The model under review builds one solid part; all positions refer to its coordinate system, in mm. Face numbers are marked on the shaded views. Coordinates: 2 decimals unless noted, no trailing zeros. Write each loop counter-clockwise with the first axis right and the second up, starting at its lowest first coordinate (ties: lowest second). Pieces come first, ordered by that corner, then holes. Notation, with made-up numbers: (9.25, -23.75) - (59.25, -23.75) arc R7 cw to (59.25, -15.75) - close; hole circle Ø5 at (55, 87). An arc over 180 degrees is marked (long way). Use one line per item in the form item = value. Start each with the question number.
```python
from build123d import *

# Parameters (mm, degrees)
SKETCH1_R                       = 62
BOSS_EXTRUDE1_DEPTH             = 15
M4_CLEARANCE_HOLE1_D            = 4.5
M12_CLEARANCE_HOLE1_D           = 13.5
M5_TAPPED_HOLE1_D               = 4.2
M5_TAPPED_HOLE1_DEPTH           = 12.4
M5_TAPPED_HOLE1_TIP             = 1.2618073
M5_TAPPED_HOLE1_ON_FACE_2_D     = 4.2
M5_TAPPED_HOLE1_ON_FACE_2_DEPTH = 12.4
M5_TAPPED_HOLE1_ON_FACE_2_TIP   = 1.2618073
M5_TAPPED_HOLE1_ON_FACE_3_D     = 4.2
M5_TAPPED_HOLE1_ON_FACE_3_DEPTH = 12.4
M5_TAPPED_HOLE1_ON_FACE_3_TIP   = 1.2618073
M5_TAPPED_HOLE1_ON_FACE_4_D     = 4.2
M5_TAPPED_HOLE1_ON_FACE_4_DEPTH = 12.4
M5_TAPPED_HOLE1_ON_FACE_4_TIP   = 1.2618073
M5_TAPPED_HOLE1_ON_FACE_5_D     = 4.2
M5_TAPPED_HOLE1_ON_FACE_5_DEPTH = 12.4
M5_TAPPED_HOLE1_ON_FACE_5_TIP   = 1.2618073


with BuildPart() as part:
    # Sketch1 → Boss-Extrude1 (new body)
    with BuildSketch(Plane.XY):
        Circle(SKETCH1_R)
    extrude(amount=BOSS_EXTRUDE1_DEPTH)

    # M4 Clearance Hole1 (through all)
    with Locations(Plane(origin=(0, 0, 0), x_dir=(-1, 0, 0), z_dir=(0, 0, -1))):
        with Locations((-42.868257487, 24.75), (-42.868257487, -24.75), (42.868257487, -24.75), (42.868257487, 24.75)):
            Hole(M4_CLEARANCE_HOLE1_D / 2)

    # M12 Clearance Hole1 (through all)
    with Locations(Plane(origin=(0, 0, 0), x_dir=(-1, 0, 0), z_dir=(0, 0, -1))):
        with Locations((0, 0)):
            Hole(M12_CLEARANCE_HOLE1_D / 2)

    # M5 Tapped Hole1
    with Locations(Plane(origin=(0, 62, 7.5), x_dir=(1, 0, 0), z_dir=(0, 1, 0))):
        with Locations((0, 0)):
            Hole(M5_TAPPED_HOLE1_D / 2, depth=M5_TAPPED_HOLE1_DEPTH)
            with Locations((0, 0, -(M5_TAPPED_HOLE1_DEPTH + M5_TAPPED_HOLE1_TIP / 2))):  # 118° drill point
                Cone(0, M5_TAPPED_HOLE1_D / 2, M5_TAPPED_HOLE1_TIP, mode=Mode.SUBTRACT)

    # M5 Tapped Hole1 on face 2
    with Locations(Plane(origin=(58.96550401, 19.159053651, 7.5), x_dir=(-0.309016857306, 0.951056560832, 0), z_dir=(0.951056560832, 0.309016857306, 0))):
        with Locations((0, 0)):
            Hole(M5_TAPPED_HOLE1_ON_FACE_2_D / 2, depth=M5_TAPPED_HOLE1_ON_FACE_2_DEPTH)
            with Locations((0, 0, -(M5_TAPPED_HOLE1_ON_FACE_2_DEPTH + M5_TAPPED_HOLE1_ON_FACE_2_TIP / 2))):  # 118° drill point
                Cone(0, M5_TAPPED_HOLE1_ON_FACE_2_D / 2, M5_TAPPED_HOLE1_ON_FACE_2_TIP, mode=Mode.SUBTRACT)

    # M5 Tapped Hole1 on face 3
    with Locations(Plane(origin=(36.442685642, -50.159053651, 7.5), x_dir=(-0.809017116291, -0.58778508449, 0), z_dir=(0.58778508449, -0.809017116291, 0))):
        with Locations((0, 0)):
            Hole(M5_TAPPED_HOLE1_ON_FACE_3_D / 2, depth=M5_TAPPED_HOLE1_ON_FACE_3_DEPTH)
            with Locations((0, 0, -(M5_TAPPED_HOLE1_ON_FACE_3_DEPTH + M5_TAPPED_HOLE1_ON_FACE_3_TIP / 2))):  # 118° drill point
                Cone(0, M5_TAPPED_HOLE1_ON_FACE_3_D / 2, M5_TAPPED_HOLE1_ON_FACE_3_TIP, mode=Mode.SUBTRACT)

    # M5 Tapped Hole1 on face 4
    with Locations(Plane(origin=(-36.442685642, -50.159053651, 7.5), x_dir=(-0.809017116291, 0.58778508449, 0), z_dir=(-0.58778508449, -0.809017116291, 0))):
        with Locations((0, 0)):
            Hole(M5_TAPPED_HOLE1_ON_FACE_4_D / 2, depth=M5_TAPPED_HOLE1_ON_FACE_4_DEPTH)
            with Locations((0, 0, -(M5_TAPPED_HOLE1_ON_FACE_4_DEPTH + M5_TAPPED_HOLE1_ON_FACE_4_TIP / 2))):  # 118° drill point
                Cone(0, M5_TAPPED_HOLE1_ON_FACE_4_D / 2, M5_TAPPED_HOLE1_ON_FACE_4_TIP, mode=Mode.SUBTRACT)

    # M5 Tapped Hole1 on face 5
    with Locations(Plane(origin=(-58.96550401, 19.159053651, 7.5), x_dir=(-0.309016857306, -0.951056560832, 0), z_dir=(-0.951056560832, 0.309016857306, 0))):
        with Locations((0, 0)):
            Hole(M5_TAPPED_HOLE1_ON_FACE_5_D / 2, depth=M5_TAPPED_HOLE1_ON_FACE_5_DEPTH)
            with Locations((0, 0, -(M5_TAPPED_HOLE1_ON_FACE_5_DEPTH + M5_TAPPED_HOLE1_ON_FACE_5_TIP / 2))):  # 118° drill point
                Cone(0, M5_TAPPED_HOLE1_ON_FACE_5_D / 2, M5_TAPPED_HOLE1_ON_FACE_5_TIP, mode=Mode.SUBTRACT)


solid = part.part
```
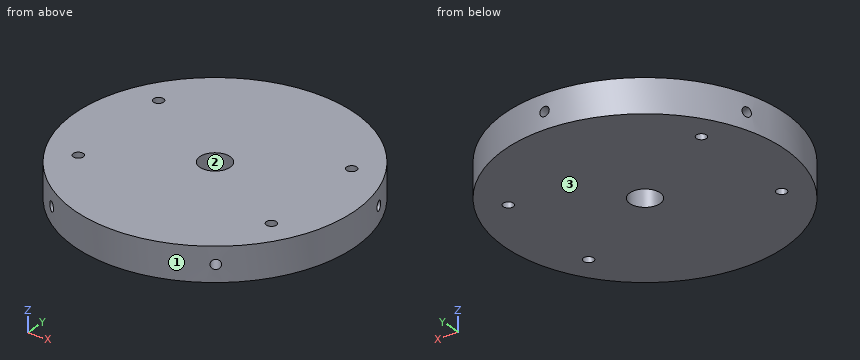
1. For L1, parallel to X at y = -42.5, z = 6.75; L2, parallel to Y at x = -49, z = 7; L3, parallel to Y at x = -50.5, z = 8.5, list the stretches that pass through material, from the lowest coordinate up.
2. For P1, Ø1, axis at x = 47, z = 8.5, coming from the +Y side; P2, Ø3, axis at y = 18, z = 2, coming from the -X side, all flat-tipped, find the tip position at first contact; note any pin that passes through.
3. Take a section at D-D (x = -11.5). State the section outline as (y, z) points, plus the area to 3 significant figures.
4. Take a section at A-A (y = 0). State the section outline as (x, z) points.
5. The part is to be moulded in two halves that separate along Y. For the marked faces 1, 2 and 3, say which applies: released by +Y, released by -Y, zero draft, split by the parting line, or undercut.
6. Take a section at B-B (y = -24.75). State the section outline as (x, z) points, plus the area to 3 significant figures.
7. Take a section at C-C (z = 11.75). State the section outline as (x, y) points, plus the area to 3 significant figures.
Returned:
q1.L1 = -45.14 to -33.3, -28.45 to 28.45, 33.3 to 45.14
q1.L2 = -37.99 to 13.78, 18.07 to 37.99
q1.L3 = -35.97 to 14.47, 18.35 to 35.97
q2.P1 = 41.01
q2.P2 = -59.76
q3.outline = (-60.92, 0) - (60.92, 0) - (60.92, 15) - (-60.92, 15) - close
q3.area = 1,830 mm²
q4.outline = (-62, 0) - (-6.75, 0) - (-6.75, 15) - (-62, 15) - close; (6.75, 0) - (62, 0) - (62, 15) - (6.75, 15) - close
q5.face_1 = split by the parting line
q5.face_2 = undercut
q5.face_3 = zero draft
q6.outline = (-56.85, 0) - (-45.12, 0) - (-45.12, 15) - (-56.85, 15) - close; (-40.62, 0) - (40.62, 0) - (40.62, 15) - (-40.62, 15) - close; (45.12, 0) - (56.85, 0) - (56.85, 15) - (45.12, 15) - close
q6.area = 1,570 mm²
q7.outline = circle Ø124 at (0, 0); hole circle Ø4.5 at (-42.87, -24.75); hole circle Ø4.5 at (-42.87, 24.75); hole circle Ø13.5 at (0, 0); hole circle Ø4.5 at (42.87, -24.75); hole circle Ø4.5 at (42.87, 24.75)
q7.area = 11,900 mm²
